Design review of the part built by this model. Coordinates are the model's own, in mm. A direction names the side the tool comes from. Coordinates: 2 decimals unless noted, no trailing zeros. Loops run counter-clockwise (first coordinate to the right, second up) from the corner with the lowest first, then second, coordinate; pieces in that order, holes last. Notation, with made-up numbers: M 15,77.5 L 68,77.5 A18 ccw 68,101.5 Z; hole C 66.5,25 d8. An arc over 180 degrees is marked long. Put each result on its own line as item: value. Start each with the question number.
(1) The part is to be moulded in two halves that separate along Y. For faces 5 (the flat face through (0, -0.5, 0)), 6 (the cylindrical face through (9.9, 1.5, 10)), 7 (the flat face through (0, -2, 0)), say which applies: +Y half, -Y half, draft (parallel to the pull), parting line (faces both ways), or undercut.
(2) Take a section at A-A, the plane y = -1.2. Give the boundary of the cut face in (x, z), then the cut area to 3 significant figures.
(3) Clearance check with flat-ended pins moving along their axes: pin 1 (1.5 mm diameter, centred on x = 4.5, z = 6, fed in from -Y); pin 2 (0.7 mm diameter, centred on x = 12, y = 3.5, fed in from +Z); pin 3 (2 mm diameter, centred on y = 2, z = 5, fed in from +X). State where each tip first meets the part, or that it passes through.
(4) For probe 1 along Y at (x, z) = (4, 1.5); probe 2 along Z at (x, y) = (1.75, 2.45), list the stretches that pass through material, from the lowest coordinate up. Write a range as [from, to].
(5) For faces 1 (the flat face through (-4.5, -1.7, -0.1)), 2 (the flat face through (0, 1, 12)), 3 (the flat face through (0, -1, -4)), 4 (the flat face through (12, 1, 0)), list the 3-axis set-ups (+Z, -Z, +X, -X, +Y, -Y) from which the entire face can be reached by the end or side of a thin tool; tool diameter is ignored.
(6) Take a section at D-D, the plane y = 1.45. Give the boundary of the cut face in (x, z).
Autodesk Inventor part; units mm, degrees
ref_plane "YZ Plane" through (0, 0, 0) normal (1, 0, 0) x (0, 1, 0)
ref_plane "XZ Plane" through (0, 0, 0) normal (0, 1, 0) x (-1, 0, 0)
ref_plane "XY Plane" through (0, 0, 0) normal (0, 0, 1) x (1, 0, 0)
sketch "스케치1" plane through (0, 0, 0) normal (0, 1, 0) x (-1, 0, 0)
  line L0 (12, 12) -> (-12, 12)
  line L1 (-12, 12) -> (-12, -12)
  line L2 (-12, -12) -> (12, -12)
  line L3 (12, -12) -> (12, 12)
  point P0 (0, 0)
  dimension "d0" = 24
  dimension "d1" = 24
  dimension "d2" = 12
  dimension "d3" = 12
extrude "돌출1" add sketch "스케치1" along normal blind 3
fillet "모깎기1" radius 7 4 edges at (-12, 1.5, 12) (12, 1.5, 12) (12, 1.5, -12) (-12, 1.5, -12)
sketch "스케치2" plane through (0, 3, 0) normal (0, 1, 0) x (1, 0, 0)
  line L0 (12.5, -4.5) -> (-12.5, -4.5)
  line L1 (-12.5, -4.5) -> (-12.5, 4.5)
  line L2 (-12.5, 4.5) -> (12.5, 4.5)
  line L3 (12.5, 4.5) -> (12.5, -4.5)
  line L4 (4.5, -12.5) -> (-4.5, -12.5)
  line L5 (-4.5, -12.5) -> (-4.5, 12.5)
  line L6 (-4.5, 12.5) -> (4.5, 12.5)
  line L7 (4.5, 12.5) -> (4.5, -12.5)
  point P0 (0, 0)
  point P1 (-4.5, -4.5)
  point P2 (-4.5, 4.5)
  point P3 (4.5, -4.5)
  point P4 (4.5, 4.5)
  dimension "d7" = 25
  dimension "d8" = 9
  dimension "d9" = 4.5
  dimension "d10" = 12.5
  dimension "d11" = 9
  dimension "d12" = 25
  dimension "d13" = 12.5
  dimension "d14" = 4.5
extrude "돌출2" add sketch "스케치2" along normal blind 0.6 contours L0 L7 L2 L3 | L7 L4 L5 L0 | L0 L1 L2 L5 | L2 L5 L6 L7
fillet "모깎기2" radius 0.6 4 edges at (12.5, 3.6, 0) (0, 3.6, -12.5) (-12.5, 3.6, 0) (0, 3.6, 12.5)
sketch "스케치3" plane through (0, 3.6, 0) normal (0, 1, 0) x (1, 0, 0)
  line L0 (11, -11) -> (-11, -11)
  line L1 (-11, -11) -> (-11, 11)
  line L2 (-11, 11) -> (11, 11)
  line L3 (11, 11) -> (11, -11)
  point P0 (0, 0)
  dimension "d18" = 22
  dimension "d19" = 22
  dimension "d20" = 11
  dimension "d21" = 11
extrude "돌출3" cut sketch "스케치3" against normal blind 0.6
sketch "스케치4" plane through (0, 0, 0) normal (0, -1, 0) x (1, 0, 0)
  line L0 (-4.5, 4.5) -> (4.5, 4.5)
  line L1 (4.5, 4.5) -> (4.5, -4.5)
  line L2 (4.5, -4.5) -> (-4.5, -4.5)
  line L3 (-4.5, -4.5) -> (-4.5, 4.5)
  point P0 (0, 0)
  dimension "d24" = 9
  dimension "d25" = 9
  dimension "d26" = 4.5
  dimension "d27" = 4.5
extrude "돌출4" add sketch "스케치4" along normal blind 2
sketch "스케치5" plane through (4.5, 0, 4.5) normal (1, 0, 0) x (0, 0, -1)
  line L0 (0.5, -1.5) -> (8.5, -1.5)
  line L1 (8.5, -1.5) -> (8.5, -0.5)
  line L2 (8.5, -0.5) -> (0.5, -0.5)
  line L3 (0.5, -0.5) -> (0.5, -1.5)
  line L4 (0, 0) -> (0, -2)
  line L5 (9, -2) -> (0, -2)
  point P0 (4.5, 0)
  dimension "d30" = 8
  dimension "d31" = 1
  dimension "d32" = 0.5
  dimension "d33" = 0.5
extrude "돌출5" cut sketch "스케치5" against normal through all
properties part number "moving_switch(bottom"
Computed values:
1. face 5: undercut
1. face 6: draft
1. face 7: -Y half
2. outline: M -4.5,-4.5 L 4.5,-4.5 L 4.5,-4 L -4.5,-4 Z; M -4.5,4 L 4.5,4 L 4.5,4.5 L -4.5,4.5 Z
2. area: 9.00 mm^2
3. pin 1: stops at y = 0
3. pin 2: stops at z = 4.5
3. pin 3: stops at x = 12
4. probe 1: y = [-2, -1.5], [-0.5, 3]
4. probe 2: z = [-12, 12]
5. face 1: +Z, -Z, -X, -Y
5. face 2: +Z, +X, -X, -Y
5. face 3: +X, -X
5. face 4: +Z, -Z, +X, -Y
6. outline: M -12,-5 A7 ccw -5,-12 L 5,-12 A7 ccw 12,-5 L 12,5 A7 ccw 5,12 L -5,12 A7 ccw -12,5 Z
